Check sheet for the drawn part. Datum: minimum x, y, z corner. Units: mm. A direction names the side the tool comes from. Round coordinates to 2 decimals unless told otherwise and drop trailing zeros. Write each loop counter-clockwise with the first axis right and the second up, starting at its lowest first coordinate (ties: lowest second). Pieces come first, ordered by that corner, then holes.
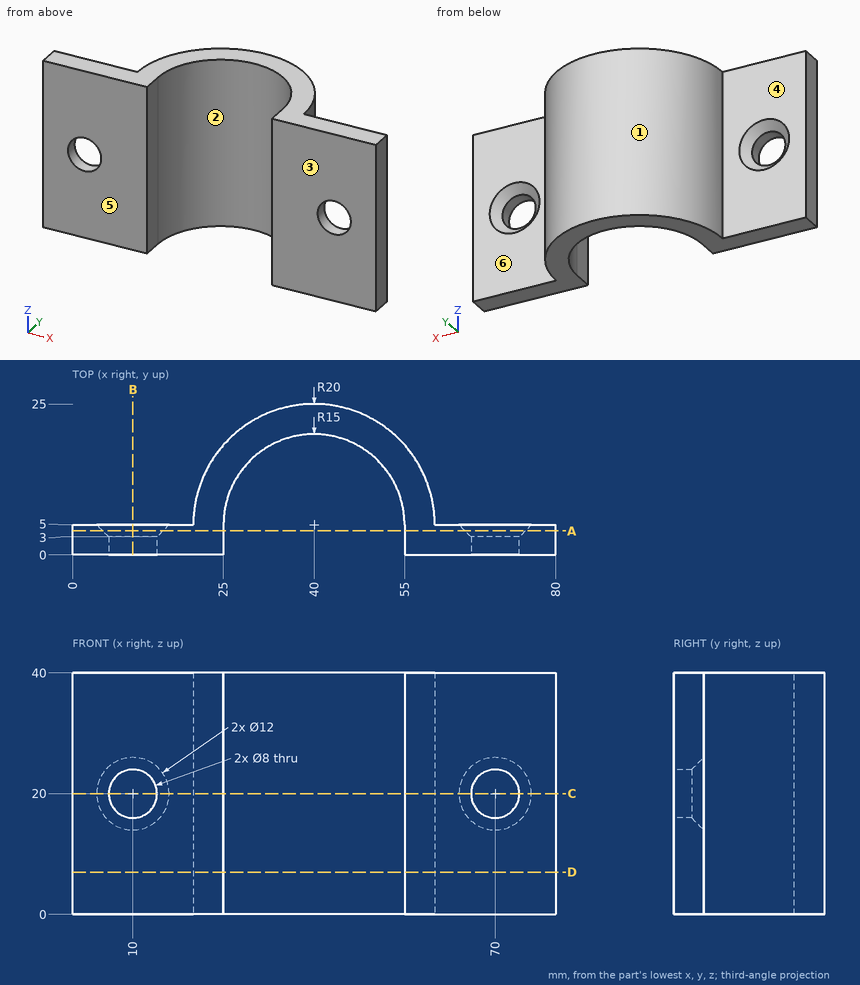
Q1. Sectioned sample at A-A (y = 4). Enter the section's corners in (x, z).
Recorded:
outline: (0, 0) - (25, 0) - (25, 40) - (0, 40) - close; (55, 0) - (80, 0) - (80, 40) - (55, 40) - close; hole circle Ø10 at (10, 20); hole circle Ø10 at (70, 20)
Q2. Material ranges on line 1 along X through (y, z) = (5.25, 4); line 2 along X through (y, z) = (3.25, 9.5); line 3 along Y through (x, z) = (67, 36.5), recorded low to high.
Recorded:
line 1: x = 20 to 25, 55 to 60
line 2: x = 0 to 25, 55 to 80
line 3: y = 0 to 5
Q3. Sectioned sample at D-D (z = 7). Enter the section's corners in (x, y).
Recorded:
outline: (0, 0) - (25, 0) - (25, 5) arc R15 cw to (55, 5) - (55, 0) - (80, 0) - (80, 5) - (60, 5) arc R20 ccw to (20, 5) - (0, 5) - close
Q4. Release check for a two-part mould opening along X. For the marked faces 1, 2 and 3 record: released by +X, released by -X, zero draft, split by the parting line, or undercut.
Recorded:
face 1: split by the parting line
face 2: undercut
face 3: zero draft
Q5. Tool access check on the marked faces 4, 5 and 6. Record the directions out of +Z, -Z, +X, -X, +Y, -Y that give a thin tool (end or side, any length) a straight path to the whole face; none if there is none.
Recorded:
face 4: +Z, -Z, -X, +Y
face 5: +Z, -Z, +X, -X, -Y
face 6: +Z, -Z, +X, +Y
Q6. Depth check by flat-ended pin: P1, Ø12, axis at y = 16.5, z = 22, coming from the -X side; P2, Ø10, axis at x = 6, z = 18.5, coming from the +Y side; P3, Ø2, axis at y = 11.5, z = 19, coming from the +X side. Enter the tip coordinate at first touch or a pass-through.
Recorded:
P1: stops at x = 20.77
P2: stops at y = 5
P3: stops at x = 59.23
Q7. Sectioned sample at C-C (z = 20). Enter the section's corners in (x, y).
Recorded:
outline: (0, 0) - (6, 0) - (6, 3) - (4, 5) - (0, 5) - close; (14, 0) - (25, 0) - (25, 5) arc R15 cw to (55, 5) - (55, 0) - (66, 0) - (66, 3) - (64, 5) - (60, 5) arc R20 ccw to (20, 5) - (16, 5) - (14, 3) - close; (74, 0) - (80, 0) - (80, 5) - (76, 5) - (74, 3) - close
Q8. Sectioned sample at B-B (x = 10). Enter the section's corners in (y, z), plus the area to 3 significant figures.
Recorded:
outline: (0, 0) - (5, 0) - (5, 14) - (3, 16) - (0, 16) - close; (0, 24) - (3, 24) - (5, 26) - (5, 40) - (0, 40) - close
area: 156 mm2
